Design review of the part built by this model. Coordinates are the model's own, in mm. Give positions to 0.01 mm unless a question says otherwise; leave off trailing zeros. Write each loop counter-clockwise with the first axis right and the second up, starting at its lowest first coordinate (ties: lowest second). Pieces come first, ordered by that corner, then holes. Notation, with made-up numbers: (13, 53.5) -> (23, 53.5) arc R13 ccw to (23, 68.5) -> close; hole circle Ø10 at (-33, -14). An arc over 180 degrees is marked (long way). Answer as a JSON object with one key per item and string values.
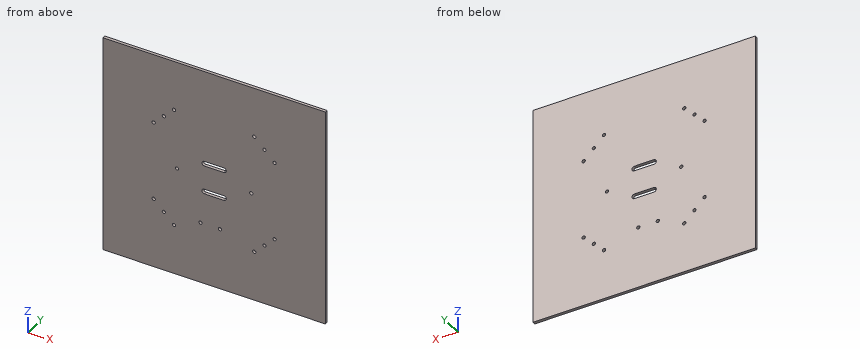
```python
from build123d import *

# Parameters (mm, degrees)
SKETCH1_W                                   = 228.6
SKETCH1_H                                   = 228.6
PLATE_DEPTH                                 = 3
SKETCH8_R                                   = 1.7
MOTOR_MOUNT_HOLES_DEPTH                     = 3
SKETCH9_R                                   = 1.7
CONNECTOR_BOARD_HOLES_DEPTH                 = 3
MOTOR_CONTROLLER_HOLDER_ARDUINO_HOLES_REACH = 163.672
SKETCH11_R                                  = 1.7
CABLE_SLOTS_REACH                           = 163.672


with BuildPart() as part:
    # Sketch1 → plate (new body)
    with BuildSketch(Plane(origin=(0, 0, 0), x_dir=(1, 0, 0), z_dir=(0, 1, 0))):
        Rectangle(SKETCH1_W, SKETCH1_H)
    extrude(amount=PLATE_DEPTH)

    # Sketch8 → motor-mount-holes (cut)
    with BuildSketch(Plane(origin=(0, 3, 0), x_dir=(1, 0, 0), z_dir=(0, 1, 0))):
        with Locations(Location((51.618795027, 51.618795027, 0), (0, 0, 270))):
            Circle(SKETCH8_R)
        with Locations(Location((62.083975388, 41.153614665, 0), (0, 0, 270))):
            Circle(SKETCH8_R)
        with Locations(Location((41.153614665, 62.083975388, 0), (0, 0, 270))):
            Circle(SKETCH8_R)
        with Locations(Location((51.618795027, -51.618795027, 0), (0, 0, 270))):
            Circle(SKETCH8_R)
        with Locations(Location((62.083975388, -41.153614665, 0), (0, 0, 270))):
            Circle(SKETCH8_R)
        with Locations(Location((41.153614665, -62.083975388, 0), (0, 0, 270))):
            Circle(SKETCH8_R)
        with Locations(Location((-51.618795027, -51.618795027, 0), (0, 0, 270))):
            Circle(SKETCH8_R)
        with Locations(Location((-41.153614665, -62.083975388, 0), (0, 0, 270))):
            Circle(SKETCH8_R)
        with Locations(Location((-62.083975388, -41.153614665, 0), (0, 0, 270))):
            Circle(SKETCH8_R)
        with Locations(Location((-51.618795027, 51.618795027, 0), (0, 0, 270))):
            Circle(SKETCH8_R)
        with Locations(Location((-62.083975388, 41.153614665, 0), (0, 0, 270))):
            Circle(SKETCH8_R)
        with Locations(Location((-41.153614665, 62.083975388, 0), (0, 0, 270))):
            Circle(SKETCH8_R)
    extrude(amount=-MOTOR_MOUNT_HOLES_DEPTH, mode=Mode.SUBTRACT)

    # Sketch9 → connector-board-holes (cut)
    with BuildSketch(Plane(origin=(0, 3, 0), x_dir=(1, 0, 0), z_dir=(0, 1, 0))):
        with Locations(Location((-38.13, 0, 0), (0, 0, 270))):
            Circle(SKETCH9_R)
        with Locations(Location((38.13, 0, 0), (0, 0, 270))):
            Circle(SKETCH9_R)
    extrude(amount=-CONNECTOR_BOARD_HOLES_DEPTH, mode=Mode.SUBTRACT)

    # Sketch11 → motor-controller-holder-arduino-holes (cut, up to next)
    with BuildSketch(Plane(origin=(0, 3, 0), x_dir=(1, 0, 0), z_dir=(0, 1, 0)), mode=Mode.PRIVATE) as motor_controller_holder_arduino_holes_sk1:
        with Locations(Location((-14, 50, 0), (0, 0, 270))):
            Circle(SKETCH11_R)
    motor_controller_holder_arduino_holes_tool1 = extrude(motor_controller_holder_arduino_holes_sk1.sketch, amount=-MOTOR_CONTROLLER_HOLDER_ARDUINO_HOLES_REACH, mode=Mode.PRIVATE) & part.part
    # Sketch11 → motor-controller-holder-arduino-holes (cut, up to next)
    with BuildSketch(Plane(origin=(0, 3, 0), x_dir=(1, 0, 0), z_dir=(0, 1, 0)), mode=Mode.PRIVATE) as motor_controller_holder_arduino_holes_sk2:
        with Locations(Location((6, 50, 0), (0, 0, 270))):
            Circle(SKETCH11_R)
    motor_controller_holder_arduino_holes_tool2 = extrude(motor_controller_holder_arduino_holes_sk2.sketch, amount=-MOTOR_CONTROLLER_HOLDER_ARDUINO_HOLES_REACH, mode=Mode.PRIVATE) & part.part
    add(motor_controller_holder_arduino_holes_tool1.solids().sort_by_distance((-14, 3, -50))[0], mode=Mode.SUBTRACT)
    add(motor_controller_holder_arduino_holes_tool2.solids().sort_by_distance((6, 3, -50))[0], mode=Mode.SUBTRACT)

    # Sketch12 → cable-slots (cut, up to next)
    with BuildSketch(Plane(origin=(0, 3, 0), x_dir=(1, 0, 0), z_dir=(0, 1, 0)), mode=Mode.PRIVATE) as cable_slots_sk1:
        with BuildLine():
            Line((-10, 17.5), (10, 17.5))
            ThreePointArc((10, 17.5), (12.5, 15), (10, 12.5))
            Line((10, 12.5), (-10, 12.5))
            ThreePointArc((-10, 12.5), (-12.5, 15), (-10, 17.5))
        make_face()
    cable_slots_tool1 = extrude(cable_slots_sk1.sketch, amount=-CABLE_SLOTS_REACH, mode=Mode.PRIVATE) & part.part
    # Sketch12 → cable-slots (cut, up to next)
    with BuildSketch(Plane(origin=(0, 3, 0), x_dir=(1, 0, 0), z_dir=(0, 1, 0)), mode=Mode.PRIVATE) as cable_slots_sk2:
        with BuildLine():
            Line((-10, -12.5), (10, -12.5))
            ThreePointArc((10, -12.5), (12.5, -15), (10, -17.5))
            Line((10, -17.5), (-10, -17.5))
            ThreePointArc((-10, -17.5), (-12.5, -15), (-10, -12.5))
        make_face()
    cable_slots_tool2 = extrude(cable_slots_sk2.sketch, amount=-CABLE_SLOTS_REACH, mode=Mode.PRIVATE) & part.part
    add(cable_slots_tool1.solids().sort_by_distance((0, 3, -15))[0], mode=Mode.SUBTRACT)
    add(cable_slots_tool2.solids().sort_by_distance((0, 3, 15))[0], mode=Mode.SUBTRACT)


solid = part.part
```
(1) For line 1 along Z through (x, y) = (-3, 0.4); line 2 along Z through (x, y) = (-11, 1.6); line 3 along X through (y, z) = (0.85, 63.5), list the stretches that pass through material, from the lowest coordinate up.
Here are the results:
{"line 1": "z = -114.3 to -17.5, -12.5 to 12.5, 17.5 to 114.3", "line 2": "z = -114.3 to -17.29, -12.71 to 12.71, 17.29 to 114.3", "line 3": "x = -114.3 to -42.09, -40.21 to 40.21, 42.09 to 114.3"}
(2) Clearance check with a flat-ended pin moving along its axis: pin 1 (4.5 mm diameter, centred on x = -14, z = -50, fed in from -Y). State where the tip first meets the part, or that it passes through.
Here are the results:
{"pin 1": "stops at y = 0"}
(3) We need section A-A, the plane x = -2. State the section outline as (y, z) points.
Here are the results:
{"outline": "(0, -114.3) -> (3, -114.3) -> (3, -17.5) -> (0, -17.5) -> close; (0, -12.5) -> (3, -12.5) -> (3, 12.5) -> (0, 12.5) -> close; (0, 17.5) -> (3, 17.5) -> (3, 114.3) -> (0, 114.3) -> close"}
